```python
from build123d import *

# Parameters (mm, degrees)
SKETCH1_W           = 30
SKETCH1_H           = 122.5
SKETCH1_R           = 2.234949948
SKETCH1_R_2         = 2.3
BOSS_EXTRUDE1_DEPTH = 13
CUT_EXTRUDE1_DEPTH  = 5
CHAMFER1_SIZE       = 0.8
SKETCH3_R           = 4.5
CUT_EXTRUDE2_DEPTH  = 8
CHAMFER2_SIZE       = 0.8


with BuildPart() as part:
    # Sketch1 → Boss-Extrude1 (new body)
    with BuildSketch(Plane(origin=(0, 0, 0), x_dir=(1, 0, 0), z_dir=(0, 1, 0))):
        Rectangle(SKETCH1_W, SKETCH1_H)
        with Locations(Location((-8, 23.25, 0), (0, 0, 90))):
            Circle(SKETCH1_R, mode=Mode.SUBTRACT)
        with Locations(Location((8, 23.25, 0), (0, 0, 90))):
            Circle(SKETCH1_R, mode=Mode.SUBTRACT)
        with Locations(Location((8, 8.25, 0), (0, 0, 90))):
            Circle(SKETCH1_R, mode=Mode.SUBTRACT)
        with Locations(Location((8, -6.75, 0), (0, 0, 90))):
            Circle(SKETCH1_R, mode=Mode.SUBTRACT)
        with Locations(Location((8, -21.75, 0), (0, 0, 90))):
            Circle(SKETCH1_R, mode=Mode.SUBTRACT)
        with Locations(Location((8, -36.75, 0), (0, 0, 90))):
            Circle(SKETCH1_R, mode=Mode.SUBTRACT)
        with Locations(Location((-8, 8.25, 0), (0, 0, 90))):
            Circle(SKETCH1_R, mode=Mode.SUBTRACT)
        with Locations(Location((-8, -6.75, 0), (0, 0, 90))):
            Circle(SKETCH1_R, mode=Mode.SUBTRACT)
        with Locations(Location((-8, -21.75, 0), (0, 0, 90))):
            Circle(SKETCH1_R, mode=Mode.SUBTRACT)
        with Locations(Location((-8, -36.75, 0), (0, 0, 90))):
            Circle(SKETCH1_R, mode=Mode.SUBTRACT)
        with Locations(Location((0, 15.75, 0), (0, 0, 90))):
            Circle(SKETCH1_R_2, mode=Mode.SUBTRACT)
        with Locations(Location((0, 0, 0), (0, 0, 90))):
            Circle(SKETCH1_R_2, mode=Mode.SUBTRACT)
    extrude(amount=BOSS_EXTRUDE1_DEPTH)

    # Sketch2 → Cut-Extrude1 (cut)
    with BuildSketch(Plane(origin=(0, 13, 0), x_dir=(1, 0, 0), z_dir=(0, 1, 0))):
        Polygon((6.066941319, 0), (3.033470659, 5.254125305), (-3.033470659, 5.254125305), (-6.066941319, 0), (-3.033470659, -5.254125305), (3.033470659, -5.254125305), align=None)
        Polygon((6.066941319, 15.75), (3.033470659, 21.004125305), (-3.033470659, 21.004125305), (-6.066941319, 15.75), (-3.033470659, 10.495874695), (3.033470659, 10.495874695), align=None)
    extrude(amount=-CUT_EXTRUDE1_DEPTH, mode=Mode.SUBTRACT)

    # Chamfer1
    chamfer1_edges = [part.edges().sort_by_distance(p)[0] for p in [
        (-15, 0, 0),
        (15, 0, 0),
    ]]
    chamfer(chamfer1_edges, length=CHAMFER1_SIZE)

    # Sketch3 → Cut-Extrude2 (cut)
    with BuildSketch(Plane.XZ):
        with Locations(Location((8, 36.75, 0), (0, 0, 270))):
            Circle(SKETCH3_R)
        with Locations(Location((-8, 36.75, 0), (0, 0, 270))):
            Circle(SKETCH3_R)
        with Locations(Location((-8, 21.75, 0), (0, 0, 270))):
            Circle(SKETCH3_R)
        with Locations(Location((-8, 6.75, 0), (0, 0, 270))):
            Circle(SKETCH3_R)
        with Locations(Location((-8, -8.25, 0), (0, 0, 270))):
            Circle(SKETCH3_R)
        with Locations(Location((-8, -23.25, 0), (0, 0, 270))):
            Circle(SKETCH3_R)
        with Locations(Location((8, 21.75, 0), (0, 0, 270))):
            Circle(SKETCH3_R)
        with Locations(Location((8, 6.75, 0), (0, 0, 270))):
            Circle(SKETCH3_R)
        with Locations(Location((8, -8.25, 0), (0, 0, 270))):
            Circle(SKETCH3_R)
        with Locations(Location((8, -23.25, 0), (0, 0, 270))):
            Circle(SKETCH3_R)
    extrude(amount=-CUT_EXTRUDE2_DEPTH, mode=Mode.SUBTRACT)

    # Chamfer2
    chamfer2_edges = [part.edges().sort_by_distance(p)[0] for p in [
        (0, 0, -61.25),
        (0, 0, 61.25),
    ]]
    chamfer(chamfer2_edges, length=CHAMFER2_SIZE)


solid = part.part
```
Model file for the job. Use its own axes, mm. A direction names the side the tool comes from. Coordinates: 2 decimals unless noted, no trailing zeros. Loops run counter-clockwise (first coordinate to the right, second up) from the corner with the lowest first, then second, coordinate; pieces in that order, holes last. Notation, with made-up numbers: (63, 21) -> (76, 21) arc R14 ccw to (76, 43) -> close; hole circle Ø5 at (8, 79.5). An arc over 180 degrees is marked (long way). Answer as a JSON object with one key per item and string values.
Q1. 3-axis set-ups, long thin cutter, end or side, ignore diameter. For faces 1 (the cylindrical face through (-5.818, 10.465, -7.766)), 2 (the flat face through (-9, 8, 9)), 3 (the flat face through (-4.53, 10.54, -18.41)): which of +Z, -Z, +X, -X, +Y, -Y reach the whole face in a straight line?
Report:
{"face 1": "+Y, -Y", "face 2": "-Y", "face 3": "+Y"}
Q2. Pull direction Z, two halves, no side cores. Call faces 4 (the flat face through (7, 8, -21)), 5 (the flat face through (-15, 7, 1)): released by +Z, released by -Z, zero draft, split by the parting line, or undercut.
Report:
{"face 4": "undercut", "face 5": "zero draft"}
Q3. Cut at B-B (z = 21.75). List the corners of the cut face in (x, y).
Report:
{"outline": "(-15, 0.8) -> (-14.2, 0) -> (-12.5, 0) -> (-12.5, 8) -> (-10.23, 8) -> (-10.23, 13) -> (-15, 13) -> close; (-5.77, 8) -> (-3.5, 8) -> (-3.5, 0) -> (3.5, 0) -> (3.5, 8) -> (5.77, 8) -> (5.77, 13) -> (-5.77, 13) -> close; (10.23, 8) -> (12.5, 8) -> (12.5, 0) -> (14.2, 0) -> (15, 0.8) -> (15, 13) -> (10.23, 13) -> close"}
Q4. Flat gauge pins, fed straight in: P1, Ø2.5, axis at x = 8.5, z = 7.5, coming from the -Y side; P2, Ø2.5, axis at x = -7.5, z = 38.5, coming from the -Y side. Where does each tip first touch, or does it go through?
Report:
{"P1": "passes through", "P2": "stops at y = 8"}
Q5. Probe probe 1 along X at (y, z) = (11.55, -8.25); probe 2 along X at (y, z) = (4.5, -8.25); probe 3 along Z at (x, y) = (8, 9.45). List the from-to ranges inside material, lowest first.
Report:
{"probe 1": "x = -15 to -10.23, -5.77 to 5.77, 10.23 to 15", "probe 2": "x = -15 to -12.5, -3.5 to 3.5, 12.5 to 15", "probe 3": "z = -61.25 to -25.48, -21.02 to -10.48, -6.02 to 4.52, 8.98 to 19.52, 23.98 to 34.52, 38.98 to 61.25"}
Q6. Cut at A-A (y = 4). State how many separate pieces and enclosed holes the cut face has, and give its area (3 significant figures).
Report:
{"separate pieces": "1", "enclosed holes": "12", "area": "3,010 mm2"}
Q7. Cut at C-C (x = 0). List the corners of the cut face in (y, z).
Report:
{"outline": "(0, -60.45) -> (0.8, -61.25) -> (13, -61.25) -> (13, -21) -> (8, -21) -> (8, -18.05) -> (0, -18.05) -> close; (0, -13.45) -> (8, -13.45) -> (8, -10.5) -> (13, -10.5) -> (13, -5.25) -> (8, -5.25) -> (8, -2.3) -> (0, -2.3) -> close; (0, 2.3) -> (8, 2.3) -> (8, 5.25) -> (13, 5.25) -> (13, 61.25) -> (0.8, 61.25) -> (0, 60.45) -> close"}
